```python
from build123d import *

# Parameters (mm, degrees)
SKETCH1_W            = 50.8
SKETCH1_H            = 55
SKETCH1_R            = 1.651
BOSS_EXTRUDE1_DEPTH  = 8.89
FILLET1_R            = 7.62
SKETCH2_W            = 50.8
SKETCH2_H            = 24.892
BOSS_EXTRUDE2_DEPTH  = 34.81959
FILLET2_R            = 7.62
SKETCH7_R            = 4.318
CUT_EXTRUDE4_DEPTH   = 40.946
BOSS_EXTRUDE4_START  = -7.62
BOSS_EXTRUDE4_DEPTH  = 35.56
MIRROR9_START        = -7.62
MIRROR9_COPY_1_DEPTH = 35.56
SKETCH10_W           = 6.35
SKETCH10_H           = 31.496
CUT_EXTRUDE5_DEPTH   = 40.946
FILLET4_R            = 2.54


with BuildPart() as part:
    # Sketch1 → Boss-Extrude1 (new body)
    with BuildSketch(Plane(origin=(0, 0, 0), x_dir=(0, 0, -1), z_dir=(1, 0, 0))):
        Rectangle(SKETCH1_W, SKETCH1_H)
        with Locations((-10, 20)):
            Circle(SKETCH1_R, mode=Mode.SUBTRACT)
        with Locations((10, 20)):
            Circle(SKETCH1_R, mode=Mode.SUBTRACT)
        with Locations((-10, -20)):
            Circle(SKETCH1_R, mode=Mode.SUBTRACT)
        with Locations((10, -20)):
            Circle(SKETCH1_R, mode=Mode.SUBTRACT)
    extrude(amount=BOSS_EXTRUDE1_DEPTH)

    # Fillet1
    fillet1_edges = [part.edges().sort_by_distance(p)[0] for p in [
        (4.445, 27.5, 25.4),
        (4.445, 27.5, -25.4),
        (4.445, -27.5, -25.4),
        (4.445, -27.5, 25.4),
    ]]
    fillet(fillet1_edges, radius=FILLET1_R)

    # Sketch2 → Boss-Extrude2 (add)
    with BuildSketch(Plane(origin=(8.89, 0, 0), x_dir=(0, 0, -1), z_dir=(1, 0, 0))):
        Rectangle(SKETCH2_W, SKETCH2_H)
    extrude(amount=BOSS_EXTRUDE2_DEPTH)

    # Fillet2
    fillet2_edges = [part.edges().sort_by_distance(p)[0] for p in [
        (26.299795, 12.446, 25.4),
        (26.299795, -12.446, 25.4),
        (26.299795, -12.446, -25.4),
        (26.299795, 12.446, -25.4),
    ]]
    fillet(fillet2_edges, radius=FILLET2_R)

    # Mirror6: part across plane


with BuildPart() as part_1:
    add(part.part)
    add(part.part.mirror(Plane(origin=(43.70959, 0, 0), x_dir=(0, 0, 1), z_dir=(1, 0, 0))))

    # Sketch7 → Cut-Extrude4 (cut, through all)
    with BuildSketch(Plane(origin=(0, 12.446, 0), x_dir=(1, 0, 0), z_dir=(0, 1, 0))):
        with Locations((34.18459, 8.255)):
            Circle(SKETCH7_R)
        with Locations((34.18459, -8.255)):
            Circle(SKETCH7_R)
        with Locations((53.23459, 8.255)):
            Circle(SKETCH7_R)
        with Locations((53.23459, -8.255)):
            Circle(SKETCH7_R)
    extrude(amount=-CUT_EXTRUDE4_DEPTH, mode=Mode.SUBTRACT)

    # Sketch9 → Boss-Extrude4 (add)
    with BuildSketch(Plane.XY.offset(25.4).offset(BOSS_EXTRUDE4_START)):
        with BuildLine():
            Line((10.326840979, 13.882840979), (8.89, 12.446))
            Line((8.89, 12.446), (13.208, 12.446))
            add(Edge.make_bspline(
                [(10.326840979, 13.882840979), (11.406340979, 12.803340979), (13.208, 12.446)],
                knots=[0.5, 0.5, 0.5, 1, 1, 1], degree=2))
        make_face()
        with BuildLine():
            add(Edge.make_bspline(
                [(8.89, 16.764), (9.247340979, 14.962340979), (10.326840979, 13.882840979)],
                knots=[0, 0, 0, 0.5, 0.5, 0.5], degree=2))
            Line((8.89, 16.764), (8.89, 12.446))
            Line((8.89, 12.446), (10.326840979, 13.882840979))
        make_face()
    boss_extrude4 = extrude(amount=-BOSS_EXTRUDE4_DEPTH)

    # Mirror8: Boss-Extrude4 across plane
    add(boss_extrude4.mirror(Plane.ZX))

    # Mirror9: Boss-Extrude4 across plane
    add(boss_extrude4.mirror(Plane(origin=(43.70959, 0, 0), x_dir=(0, 0, 1), z_dir=(1, 0, 0))))

    # Mirror9 copy 1 sketch → Mirror9 copy 1 (add)
    with BuildSketch(Plane(origin=(87.41918, 0, 25.4), x_dir=(-1, 0, 0), z_dir=(0, 0, 1)).offset(MIRROR9_START)):
        with BuildLine():
            Line((10.326840979, 13.882840979), (8.89, 12.446))
            Line((8.89, 12.446), (13.208, 12.446))
            add(Edge.make_bspline(
                [(10.326840979, 13.882840979), (11.406340979, 12.803340979), (13.208, 12.446)],
                knots=[0.5, 0.5, 0.5, 1, 1, 1], degree=2))
        make_face()
        with BuildLine():
            add(Edge.make_bspline(
                [(8.89, 16.764), (9.247340979, 14.962340979), (10.326840979, 13.882840979)],
                knots=[0, 0, 0, 0.5, 0.5, 0.5], degree=2))
            Line((8.89, 16.764), (8.89, 12.446))
            Line((8.89, 12.446), (10.326840979, 13.882840979))
        make_face()
    extrude(amount=-MIRROR9_COPY_1_DEPTH)

    # Sketch10 → Cut-Extrude5 (cut, through all)
    with BuildSketch(Plane(origin=(0, 12.446, 0), x_dir=(1, 0, 0), z_dir=(0, 1, 0))):
        with Locations((17.907, 0)):
            Rectangle(SKETCH10_W, SKETCH10_H)
    cut_extrude5 = extrude(amount=-CUT_EXTRUDE5_DEPTH, mode=Mode.SUBTRACT)

    # Mirror10: Cut-Extrude5 across plane
    add(cut_extrude5.mirror(Plane(origin=(43.70959, 0, 0), x_dir=(0, 0, 1), z_dir=(1, 0, 0))), mode=Mode.SUBTRACT)

    # Fillet4
    fillet4_edges = [part_1.edges().sort_by_distance(p)[0] for p in [
        (21.082, -12.446, 0),
        (21.082, 12.446, 0),
        (66.33718, 12.446, 0),
        (66.33718, -12.446, 0),
    ]]
    fillet(fillet4_edges, radius=FILLET4_R)


solid = part_1.part
```
Design review of the part built by this model. Coordinates are the model's own, in mm. A direction names the side the tool comes from. Give positions to 0.01 mm unless a question says otherwise; leave off trailing zeros. Loops run counter-clockwise (first coordinate to the right, second up) from the corner with the lowest first, then second, coordinate; pieces in that order, holes last. Notation, with made-up numbers: (-14.5, 79.5) -> (30.5, 79.5) arc R13 ccw to (30.5, 86.5) -> close; hole circle Ø5 at (54.5, 17). An arc over 180 degrees is marked (long way). One line per item, written item: value.
Q1. Draft analysis for pull direction Y (two halves, no side actions). For faces 1 (the flat face through (10, -14, 17.78)), 2 (the cylindrical face through (4.383, 18.535, -10.762)), 3 (the flat face through (4, -27.5, 0)), 4 (the flat face through (44, 12.446, 0)), state which applies: pulls with the +Y half, pulls with the -Y half, needs draft (parallel to the pull), parting line crosses it, or undercut.
Numbers:
face 1: needs draft
face 2: undercut
face 3: pulls with the -Y half
face 4: pulls with the +Y half
Q2. We need section B-B on z = 0.5. Give the number of separate pieces and of enclosed holes in the cut face, and give its area (3 significant figures).
Numbers:
separate pieces: 3
enclosed holes: 0
area: 2,410 mm^2
Q3. We need section A-A on x = 67.5. Give the boundary of the cut face in (y, z), and give its area (3 significant figures).
Numbers:
outline: (-12.45, -17.78) arc R7.62 ccw to (-4.83, -25.4) -> (4.83, -25.4) arc R7.62 ccw to (12.45, -17.78) -> (12.45, -15.75) -> (-12.45, -15.75) -> close; (-12.45, 15.75) -> (12.45, 15.75) -> (12.45, 17.78) arc R7.62 ccw to (4.83, 25.4) -> (-4.83, 25.4) arc R7.62 ccw to (-12.45, 17.78) -> close
area: 431 mm^2
Q4. We need section C-C on x = 42.5. Give the boundary of the cut face in (y, z), and give its area (3 significant figures).
Numbers:
outline: (-12.45, -17.78) arc R7.62 ccw to (-4.83, -25.4) -> (4.83, -25.4) arc R7.62 ccw to (12.45, -17.78) -> (12.45, 17.78) arc R7.62 ccw to (4.83, 25.4) -> (-4.83, 25.4) arc R7.62 ccw to (-12.45, 17.78) -> close
area: 1,210 mm^2
Q5. For pin 1 Ø3.5 at (x, y) = (11, 15.5) entering from -Z; pin 2 Ø3 at (y, z) = (20, 10) entering from +X; pin 3 Ø2 at (x, z) = (21, -14) entering from +Y; pin 4 Ø10 at (x, z) = (69, 16) entering from +Y, all flat-tipped, find the tip position at first contact; note any pin that passes through.
Numbers:
pin 1: stops at z = -17.78
pin 2: passes through
pin 3: stops at y = 11.86
pin 4: stops at y = 12.45
Q6. We need section D-D on z = -20. Give the boundary of the cut face in (x, y).
Numbers:
outline: (0, -27.17) -> (8.89, -27.17) -> (8.89, -12.12) -> (78.53, -12.12) -> (78.53, -27.17) -> (87.42, -27.17) -> (87.42, 27.17) -> (78.53, 27.17) -> (78.53, 12.12) -> (8.89, 12.12) -> (8.89, 27.17) -> (0, 27.17) -> close
Q7. Machinability: for faces 5 (the cylindrical face through (82.912, 25.209, 23.227)), 6 (the flat face through (66.337, 0, 0)), 7 (the flat face through (10, 14, -17.78)), 8 (the flat face through (0, 0, 0)), 9 (the flat face through (10, 14, 17.78)), which of the approach directions +Z, -Z, +X, -X, +Y, -Y give a long, thin tool a straight path to every point of the face, cutting with its end or side? Answer none if there is none.
Numbers:
face 5: +Z, +X, -X, +Y
face 6: +Y, -Y
face 7: -Z, +Y
face 8: +Z, -Z, -X, +Y, -Y
face 9: +Z, +Y
Q8. For L1, parallel to Y at x = 4, z = -10; L2, parallel to X at y = -21, z = 18.5; L3, parallel to Z at x = 67.5, y = -1, list the stretches that pass through material, from the lowest coordinate up.
Numbers:
L1: y = -27.5 to -21.65, -18.35 to 18.35, 21.65 to 27.5
L2: x = 0 to 8.89, 78.53 to 87.42
L3: z = -25.4 to -15.75, 15.75 to 25.4
